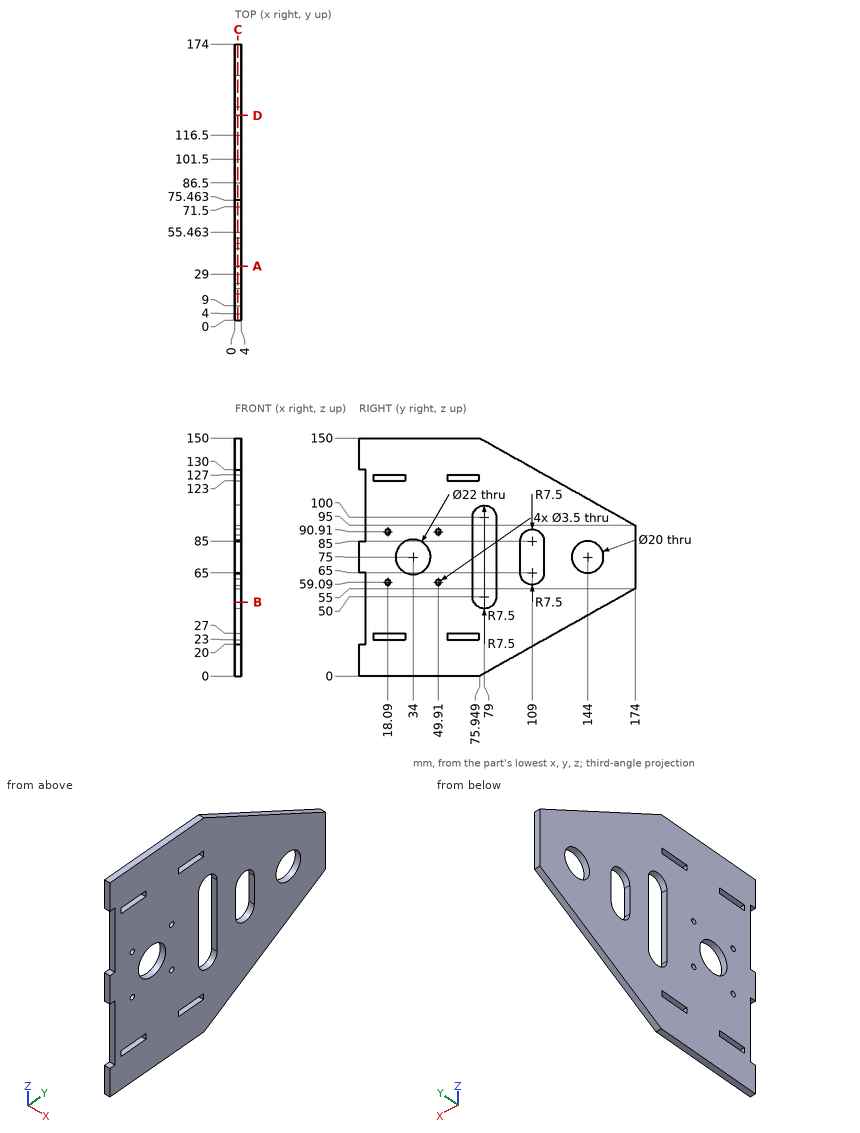
Could you check a few things on this drawing? It's one solid part, dimensions in mm from its lowest x, y, z. Coordinates: 2 decimals unless noted, no trailing zeros. Write each loop counter-clockwise with the first axis right and the second up, starting at its lowest first coordinate (ties: lowest second). Pieces come first, ordered by that corner, then holes. Notation, with made-up numbers: (75.25, 88) - (98.25, 88) arc R12 ccw to (98.25, 101) - close; hole circle Ø6 at (89.25, -3.5). An arc over 180 degrees is marked (long way). Return JSON: item names as keys, results as strings. Group by question number.
Item 1: Please list where these lines run through material, in increasing order: probe 1 along Z at (x, y) = (3.3, 65.5); probe 2 along Y at (x, z) = (0.4, 71.5); probe 3 along Y at (x, z) = (1.45, 81).
Item 2: If we section it at D-D (y = 129): Write out the boundary of the cut face in (x, z), then the cut area to 3 significant figures.
Item 3: If we section it at B-B (z = 46.5): Write out the boundary of the cut face in (x, y).
Item 4: If we section it at C-C (x = 2): Count the separate pieces of the cut face and the enclosed holes in it, then the cut area to 3 significant figures.
Item 5: If we section it at A-A (y = 34): Write out the boundary of the cut face in (x, z), then the cut area to 3 significant figures.
Item 6: I'm going to push flat-ended pins straight in: pin 1 Ø1.5 at (x, y) = (2, 132.5) entering from -Z; pin 2 Ø2 at (x, y) = (3.5, 105) entering from -Z (1 decimal); pin 3 Ø1.2 at (x, z) = (1.5, 111.5) entering from -Y. Where does each tip first touch, or does it pass through?
Return value:
{
 "1": {"probe 1": "z = 0 to 23, 27 to 123, 127 to 150", "probe 2": "y = 0 to 23.57, 44.43 to 71.5, 86.5 to 101.5, 116.5 to 134.63, 153.37 to 174", "probe 3": "y = 0 to 24.78, 43.22 to 71.5, 86.5 to 101.5, 116.5 to 136, 152 to 174"},
 "2": {"outline": "(0, 29.76) - (4, 29.76) - (4, 120.24) - (0, 120.24) - close", "area": "362 mm^2"},
 "3": {"outline": "(0, 4) - (4, 4) - (4, 72.37) - (0, 72.37) - close; (0, 85.63) - (4, 85.63) - (4, 158.85) - (0, 158.85) - close"},
 "4": {"separate pieces": "1", "enclosed holes": "12", "area": "17,900 mm^2"},
 "5": {"outline": "(0, 0) - (4, 0) - (4, 64) - (0, 64) - close; (0, 86) - (4, 86) - (4, 150) - (0, 150) - close", "area": "512 mm^2"},
 "6": {"pin 1": "stops at z = 31.3", "pin 2": "stops at z = 15.7", "pin 3": "stops at y = 4"}
}
